from build123d import *

# Parameters (mm, degrees)
SALIENTE_EXTRUIR1_DEPTH    = 4.9
SALIENTE_EXTRUIR1_TAPER    = 7
CROQUIS2_R                 = 5.8
SALIENTE_EXTRUIR2_DEPTH    = 0.3
CORTAR_EXTRUIR1_DEPTH      = 6.2
CROQUIS4_R                 = 5.8
SALIENTE_EXTRUIR3_DEPTH    = 0.3
CORTAR_EXTRUIR2_DEPTH      = 6.2
CORTAR_EXTRUIR3_DEPTH      = 3.75
CROQUIS7_W                 = 4.85
CROQUIS7_H                 = 0.9
CROQUIS8_W                 = 4.85
CROQUIS8_H                 = 0.9
CROQUIS9_W                 = 3.415
CROQUIS9_H                 = 0.3
CROQUIS10_W                = 3.415
CROQUIS10_H                = 0.3
CROQUIS11_OUTSIDE_W        = 43.344
CROQUIS11_OUTSIDE_H        = 24.694
CROQUIS11_OUTSIDE_R        = 6.99
CORTAR_EXTRUIR8_DEPTH      = 5.9000001
CORTAR_EXTRUIR8_DEPTH_BACK = 1.3
CROQUIS20_R                = 7.6
CROQUIS20_R_2              = 5.8
SALIENTE_EXTRUIR11_DEPTH   = 4.9
SALIENTE_EXTRUIR11_TAPER   = 7
REDONDEO6_R                = 0.5


with BuildPart() as part:
    # Croquis1 → Saliente-Extruir1 (new body)
    with BuildSketch(Plane.XZ):
        with BuildLine():
            Line((-9.325, -7.6), (9.325, -7.6))
            ThreePointArc((9.325, -7.6), (16.925, 0), (9.325, 7.6))
            Line((9.325, 7.6), (-9.325, 7.6))
            ThreePointArc((-9.325, 7.6), (-16.925, 0), (-9.325, -7.6))
        make_face()
    extrude(amount=-SALIENTE_EXTRUIR1_DEPTH, taper=SALIENTE_EXTRUIR1_TAPER)

    # Croquis2 → Saliente-Extruir2 (add)
    with BuildSketch(Plane.XZ):
        with Locations((9.325, 0)):
            Circle(CROQUIS2_R)
    extrude(amount=SALIENTE_EXTRUIR2_DEPTH)

    # Croquis3 → Cortar-Extruir1 (cut, through all)
    with BuildSketch(Plane(origin=(0, 4.9, 0), x_dir=(-1, 0, 0), z_dir=(0, 1, 0))):
        with BuildLine():
            Line((-10.459680572, -2.45), (-8.190319428, -2.45))
            ThreePointArc((-8.190319428, -2.45), (-6.625, 0), (-8.190319428, 2.45))
            Line((-8.190319428, 2.45), (-10.459680572, 2.45))
            ThreePointArc((-10.459680572, 2.45), (-12.025, 0), (-10.459680572, -2.45))
        make_face()
    extrude(amount=-CORTAR_EXTRUIR1_DEPTH, mode=Mode.SUBTRACT)

    # Croquis4 → Saliente-Extruir3 (add)
    with BuildSketch(Plane.XZ):
        with Locations((-9.325, 0)):
            Circle(CROQUIS4_R)
    extrude(amount=SALIENTE_EXTRUIR3_DEPTH)

    # Croquis5 → Cortar-Extruir2 (cut, through all)
    with BuildSketch(Plane(origin=(0, 4.9, 0), x_dir=(-1, 0, 0), z_dir=(0, 1, 0))):
        with BuildLine():
            Line((10.459680572, 2.45), (8.190319428, 2.45))
            ThreePointArc((8.190319428, 2.45), (6.625, 0), (8.190319428, -2.45))
            Line((8.190319428, -2.45), (10.459680572, -2.45))
            ThreePointArc((10.459680572, -2.45), (12.025, 0), (10.459680572, 2.45))
        make_face()
    extrude(amount=-CORTAR_EXTRUIR2_DEPTH, mode=Mode.SUBTRACT)

    # Croquis6 → Cortar-Extruir3 (cut)
    with BuildSketch(Plane.XZ):
        with BuildLine():
            Line((-2.15, 2.8), (-2.15, -2.8))
            ThreePointArc((-2.15, -2.8), (0, -4.95), (2.15, -2.8))
            Line((2.15, -2.8), (2.15, 2.8))
            ThreePointArc((2.15, 2.8), (0, 4.95), (-2.15, 2.8))
        make_face()
    extrude(amount=-CORTAR_EXTRUIR3_DEPTH, mode=Mode.SUBTRACT)

    # Croquis7 → Cortar-Revolución1 (revolve, cut)
    with BuildSketch(Plane(origin=(-9.325, 0, 0), x_dir=(0, 0, -1), z_dir=(1, 0, 0))):
        with Locations((2.425, 4.55)):
            Rectangle(CROQUIS7_W, CROQUIS7_H)
    revolve(axis=Axis((-9.325, 5, 0), (0, -1, 0)), mode=Mode.SUBTRACT)

    # Croquis8 → Cortar-Revolución2 (revolve, cut)
    with BuildSketch(Plane(origin=(9.325, 0, 0), x_dir=(0, 0, -1), z_dir=(1, 0, 0))):
        with Locations((2.425, 4.55)):
            Rectangle(CROQUIS8_W, CROQUIS8_H)
    revolve(axis=Axis((9.325, 5, 0), (0, -1, 0)), mode=Mode.SUBTRACT)

    # Croquis9 → Cortar-Revolución3 (revolve, cut)
    with BuildSketch(Plane(origin=(-9.325, 0, 0), x_dir=(0, 0, -1), z_dir=(1, 0, 0))):
        with Locations((1.7075, -0.15)):
            Rectangle(CROQUIS9_W, CROQUIS9_H)
    revolve(axis=Axis((-9.325, 0, 0), (0, -1, 0)), mode=Mode.SUBTRACT)

    # Croquis10 → Cortar-Revolución4 (revolve, cut)
    with BuildSketch(Plane(origin=(9.325, 0, 0), x_dir=(0, 0, -1), z_dir=(1, 0, 0))):
        with Locations((1.7075, -0.15)):
            Rectangle(CROQUIS10_W, CROQUIS10_H)
    revolve(axis=Axis((9.325, 0, 0), (0, -1, 0)), mode=Mode.SUBTRACT)

    # Croquis11 outside → Cortar-Extruir8 (cut, two sides)
    with BuildSketch(Plane(origin=(0, 0, 0), x_dir=(1, 0, 0), z_dir=(0, 1, 0))) as cortar_extruir8_sk:
        Rectangle(CROQUIS11_OUTSIDE_W, CROQUIS11_OUTSIDE_H)
        with Locations((-9.325, 0)):
            Circle(CROQUIS11_OUTSIDE_R, mode=Mode.SUBTRACT)
    extrude(amount=CORTAR_EXTRUIR8_DEPTH, mode=Mode.SUBTRACT)
    extrude(cortar_extruir8_sk.sketch, amount=-CORTAR_EXTRUIR8_DEPTH_BACK, mode=Mode.SUBTRACT)

    # Croquis20 → Saliente-Extruir11 (add)
    with BuildSketch(Plane.XZ):
        with Locations((-9.325, 0)):
            Circle(CROQUIS20_R)
        with Locations((-9.325, 0)):
            Circle(CROQUIS20_R_2, mode=Mode.SUBTRACT)
    extrude(amount=-SALIENTE_EXTRUIR11_DEPTH, taper=SALIENTE_EXTRUIR11_TAPER)

    # Redondeo6
    redondeo6_edges = [part.edges().sort_by_distance(p)[0] for p in [
        (-16.323355652, 4.9, 0),
    ]]
    fillet(redondeo6_edges, radius=REDONDEO6_R)


solid = part.part
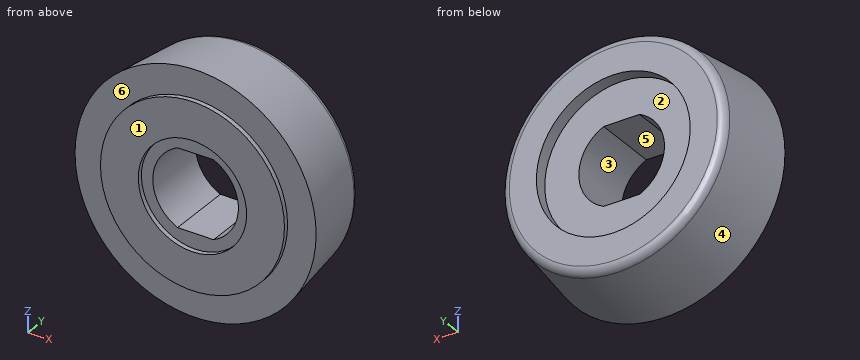
Check sheet for the modelled part. Datum: model origin and axes. Units: mm. Face numbers are marked on the shaded views. A direction names the side the tool comes from. Round coordinates to 2 decimals unless told otherwise and drop trailing zeros. Write each loop counter-clockwise with the first axis right and the second up, starting at its lowest first coordinate (ties: lowest second). Pieces come first, ordered by that corner, then holes. Notation, with made-up numbers: (-23.75, 52.5) - (18.25, 52.5) arc R36 cw to (18.25, 87.5) - close; hole circle Ø11 at (-34.75, 65.5). An arc over 180 degrees is marked (long way). Return JSON: item names as keys, results as strings.
Q1. Draft check along X on the marked faces 4, 5 and 6. Enter one of: released by +X, released by -X, zero draft, split by the parting line, or undercut.
Returned:
{"face 4": "split by the parting line", "face 5": "undercut", "face 6": "zero draft"}
Q2. Cross-section at B-B (y = 2.15). Record the boundary of the cut face in (x, z) (3 decimals).
Returned:
{"outline": "circle Ø14.672 at (-9.325, 0); hole (-10.46, -2.45) - (-8.19, -2.45) arc R2.7 ccw to (-8.19, 2.45) - (-10.46, 2.45) arc R2.7 ccw to start"}
Q3. Scan lines: L1, parallel to Y at x = -6, z = -3; L2, parallel to Z at x = -10.5, y = 3.3; L3, parallel to X at y = 1.6, z = 1. Record each from-to range of solid material in increasing order. Write a range as from..to.
Returned:
{"L1": "y = -0.3..4.1", "L2": "z = -7.1..-2.43, 2.43..7.1", "L3": "x = -16.66..-11.83, -6.82..-1.99"}
Q4. Cross-section at A-A (y = 0.95). Record the boundary of the cut face in (x, z) (3 decimals), then the cut area to 3 significant figures.
Returned:
{"outline": "circle Ø14.967 at (-9.325, 0); hole (-10.46, -2.45) - (-8.19, -2.45) arc R2.7 ccw to (-8.19, 2.45) - (-10.46, 2.45) arc R2.7 ccw to start", "area": "154 mm²"}
Q5. Depth check by flat-ended pin: P1, Ø2, axis at x = -10, z = -3.5, coming from the +Y side; P2, Ø1.1, axis at x = -9, y = 1.5, coming from the -Z side; P3, Ø1.8, axis at x = -9, y = 2.5, coming from the +Z side. Enter the tip coordinate at first touch or a pass-through.
Returned:
{"P1": "stops at y = 4.1", "P2": "stops at z = -7.48", "P3": "stops at z = 7.4"}
Q6. Access from +Z, -Z, +X, -X, +Y, -Y to the whole of each face (thin tool, end or side, straight path). Record for the marked faces 1, 2 and 3.
Returned:
{"face 1": "+Z, -Z, +X, -X, -Y", "face 2": "+Y", "face 3": "+Y, -Y"}
